Geometry check sheet. Reference: the model listing, model coordinates, mm. Round coordinates to 2 decimals unless told otherwise and drop trailing zeros. Order: outer loops, then holes, each group sorted by start corner. A loop starts at its lowest first (then second) coordinate and runs counter-clockwise, first axis right, second up.
```python
from build123d import *

# Parameters (mm, degrees)
SKETCH1_W           = 15
SKETCH1_H           = 15
SKETCH1_W_2         = 14
SKETCH1_H_2         = 14
BOSS_EXTRUDE1_DEPTH = 165
FILLET1_R           = 2
SKETCH2_R           = 2
CUT_EXTRUDE2_DEPTH  = 28


with BuildPart() as part:
    # Sketch1 → Boss-Extrude1 (new body)
    with BuildSketch(Plane.XY):
        Rectangle(SKETCH1_W, SKETCH1_H)
        Rectangle(SKETCH1_W_2, SKETCH1_H_2, mode=Mode.SUBTRACT)
    extrude(amount=BOSS_EXTRUDE1_DEPTH)

    # Fillet1
    fillet1_edges = [part.edges().sort_by_distance(p)[0] for p in [
        (-7, 7, 82.5),
        (-7, -7, 82.5),
        (7, -7, 82.5),
        (7, 7, 82.5),
        (-7.5, 7.5, 82.5),
        (7.5, 7.5, 82.5),
        (7.5, -7.5, 82.5),
        (-7.5, -7.5, 82.5),
    ]]
    fillet(fillet1_edges, radius=FILLET1_R)

    # Sketch2 → Cut-Extrude2 (cut)
    with BuildSketch(Plane.XZ.offset(7.5)):
        with Locations((0, 162)):
            Circle(SKETCH2_R)
        with Locations((0, 138)):
            Circle(SKETCH2_R)
        with Locations((0, 27)):
            Circle(SKETCH2_R)
        with Locations((0, 3)):
            Circle(SKETCH2_R)
    extrude(amount=-CUT_EXTRUDE2_DEPTH, mode=Mode.SUBTRACT)


solid = part.part
```
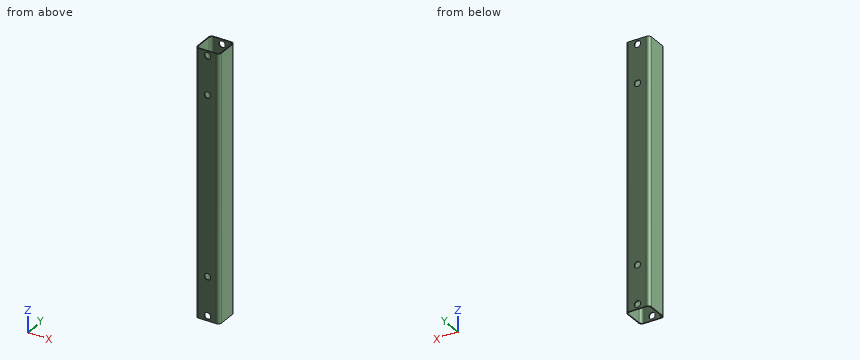
(1) Material ranges on line 1 (Z direction, x = 0, y = 7.45); line 2 (X direction, y = 0, z = 129.5), recorded low to high.
Returned:
line 1: z = 0 to 1, 5 to 25, 29 to 136, 140 to 160, 164 to 165
line 2: x = -7.5 to -7, 7 to 7.5
(2) Depth check by flat-ended pin: P1, Ø3.5, axis at x = 0, z = 162, coming from the +Y side. Enter the tip coordinate at first touch or a pass-through.
Returned:
P1: passes through
(3) Sectioned sample at D-D, the plane x = 0. Give the number of separate pieces and of enclosed holes in the cut face, and give its area (3 significant figures).
Returned:
separate pieces: 10
enclosed holes: 0
area: 149 mm2
(4) Sectioned sample at B-B, the plane y = 1. Record the cut outline in (x, z), and give its area (3 significant figures).
Returned:
outline: (-7.5, 0) - (-7, 0) - (-7, 165) - (-7.5, 165) - close; (7, 0) - (7.5, 0) - (7.5, 165) - (7, 165) - close
area: 165 mm2
(5) Sectioned sample at A-A, the plane z = 162. Record the cut outline in (x, y).
Returned:
outline: (-7.5, -5.5) arc R2 ccw to (-5.5, -7.5) - (-2, -7.5) - (-2, -7) - (-5, -7) arc R2 cw to (-7, -5) - (-7, 5) arc R2 cw to (-5, 7) - (-2, 7) - (-2, 7.5) - (-5.5, 7.5) arc R2 ccw to (-7.5, 5.5) - close; (2, -7.5) - (5.5, -7.5) arc R2 ccw to (7.5, -5.5) - (7.5, 5.5) arc R2 ccw to (5.5, 7.5) - (2, 7.5) - (2, 7) - (5, 7) arc R2 cw to (7, 5) - (7, -5) arc R2 cw to (5, -7) - (2, -7) - close
(6) Sectioned sample at C-C, the plane z = 58. Record the cut outline in (x, y).
Returned:
outline: (-7.5, -5.5) arc R2 ccw to (-5.5, -7.5) - (5.5, -7.5) arc R2 ccw to (7.5, -5.5) - (7.5, 5.5) arc R2 ccw to (5.5, 7.5) - (-5.5, 7.5) arc R2 ccw to (-7.5, 5.5) - close; hole (-7, -5) arc R2 ccw to (-5, -7) - (5, -7) arc R2 ccw to (7, -5) - (7, 5) arc R2 ccw to (5, 7) - (-5, 7) arc R2 ccw to (-7, 5) - close
